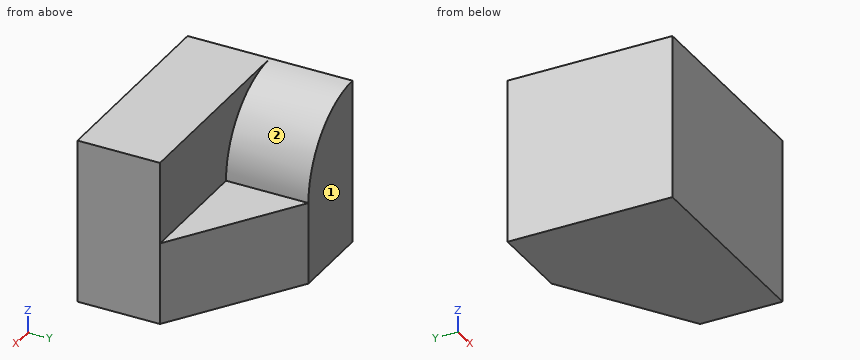
Autodesk Inventor part; units mm, degrees
ref_plane "YZ Plane" through (0, 0, 0) normal (1, 0, 0) x (0, 1, 0)
ref_plane "XZ Plane" through (0, 0, 0) normal (0, 1, 0) x (-1, 0, 0)
ref_plane "XY Plane" through (0, 0, 0) normal (0, 0, 1) x (1, 0, 0)
sketch "草圖1" plane through (0, 0, 0) normal (0, 1, 0) x (-1, 0, 0)
  line L0 (0, 0) -> (-50, 0)
  line L1 (-50, 0) -> (-50, -40)
  line L2 (-50, -40) -> (0, -40)
  line L3 (0, -40) -> (0, 0)
  dimension "d0" = 50
  dimension "d1" = 40
extrude "擠出1" add sketch "草圖1" along normal blind 20
sketch "草圖2" plane through (0, 20, 0) normal (0, 1, 0) x (1, 0, 0)
  line L0 (0, 40) -> (20, 40)
  line L1 (20, 40) -> (20, 0)
  line L2 (20, 0) -> (0, 0)
  line L3 (0, 0) -> (0, 40)
  line L4 (50, 40) -> (0, 40)
  line L5 (0, 40) -> (0, 0)
  dimension "d4" = 20
extrude "擠出2" add sketch "草圖2" along normal blind 20
fillet "圓角1" radius 20 1 edges at (20, 30, 0)
sketch "草圖3" plane through (50, 0, -40) normal (0, 0, -1) x (-1, 0, 0)
  line L0 (30, 40) -> (50, 40)
  line L1 (0, 20) -> (30, 20)
  line L2 (30, 40) -> (0, 20)
  line L3 (0, 20) -> (30, 20)
  line L4 (30, 20) -> (30, 40)
  line L5 (30, 20) -> (30, 40)
  point P0 (50, 0)
extrude "擠出3" add sketch "草圖3" against normal blind 20
properties part number "39 (60283.185 mm^3)"
Work out the finished part from the listing and answer in its coordinate system (mm). Face numbers are marked on the shaded views. A direction names the side the tool comes from. Round coordinates to 2 decimals unless told otherwise and drop trailing zeros. Loops run counter-clockwise (first coordinate to the right, second up) from the corner with the lowest first, then second, coordinate; pieces in that order, holes last. Notation, with made-up numbers: (-22.5, 32.25) - (-17.5, 32.25) arc R34 cw to (-17.5, 62.25) - close; hole circle Ø9 at (-16.75, 87). An arc over 180 degrees is marked (long way). One line per item, written item: value.
Q1. Find section B-B on z = -36. Give the vertices of the cut face in (x, y).
Check values:
outline: (0, 0) - (50, 0) - (50, 20) - (20, 40) - (0, 40) - close
Q2. Find section C-C on x = 44. Give the vertices of the cut face in (y, z).
Check values:
outline: (0, -40) - (24, -40) - (24, -20) - (20, -20) - (20, 0) - (0, 0) - close
Q3. Straight lines are drawn through the part: probe 1 along Z at (x, y) = (27, 25); probe 2 along Y at (x, z) = (36, -3.5); probe 3 along X at (y, z) = (24, -21). For each, find the intervals that lie inside material, in ascending order.
Check values:
probe 1: -40 to -20
probe 2: 0 to 20
probe 3: 0 to 44
Q4. Each of these flat-tipped pins is pushed along its axis until it touches: pin 1 Ø16 at (x, y) = (37, 27) entering from +Z; pin 2 Ø5 at (x, y) = (44.5, 26.5) entering from +Z; pin 3 Ø8 at (y, z) = (33.5, -12.5) entering from +X; pin 4 Ø1 at (y, z) = (23.5, -25) entering from +X. Where does it stop, or does it pass through?
Check values:
pin 1: z = 0
pin 2: z = -20
pin 3: x = 19.69
pin 4: x = 45.5
Q5. For the marked faces 1 and 2, determine the directions among +Z, -Z, +X, -X, +Y, -Y from which every point of the face is accessible in a straight line to the end or side of a thin tool.
Check values:
face 1: +Z, -Z, +X, -X, +Y
face 2: +Z, +X, +Y
